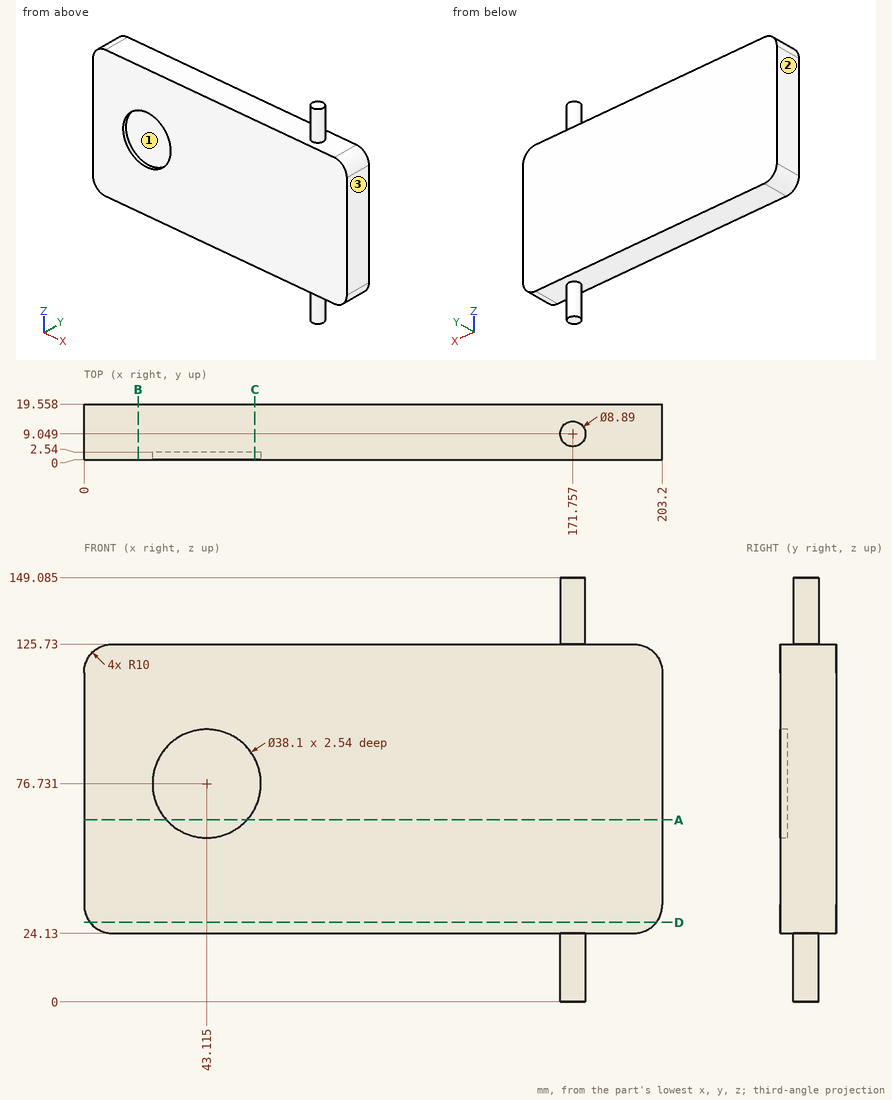
The drawing under review shows one solid part. Ordinate dimensions are in mm from its lowest x, y, z. Give positions to 0.01 mm unless a question says otherwise; leave off trailing zeros. Loops run counter-clockwise (first coordinate to the right, second up) from the corner with the lowest first, then second, coordinate; pieces in that order, holes last. Notation, with made-up numbers: M 21,-32 L 55,-32 A22 cw 55,-16 Z; hole C 88,-26 d5. An arc over 180 degrees is marked long. One line per question, with ' | ' between items. Start each with the question number.
1. To check wall thickness, follow L1, parallel to Z at x = 110, y = 8; L2, parallel to Z at x = 26, y = 2.25 (1 decimal); L3, parallel to X at y = 12.5, z = 140 (1 decimal). State the ranges of each line that lie inside material, in increasing order.
2. Add section A-A (z = 64). Write out the cut boundary in (x, y) (1 decimal).
3. Insertion check: P1, Ø6, axis at x = 109.5, y = 6.5, coming from the +Z side; P2, Ø10, axis at x = 112.5, y = 8.5, coming from the -Z side. Each pin has a flat end and moves straight along its axis. Give the tip position at first contact, or say it passes through.
4. Add section D-D (z = 28). Write out the cut boundary in (x, y), plus the area to 3 significant figures.
5. The part is to be moulded in two halves that separate along X. For the marked faces 1, 2 and 3, say which applies: released by +X, released by -X, zero draft, split by the parting line, or undercut.
6. Add section B-B (x = 19). Write out the cut boundary in (y, z).
7. Add section C-C (x = 60). Write out the cut boundary in (y, z), plus the area to 3 significant figures.
Worked out:
1) L1: z = 24.13 to 125.73 | L2: z = 24.1 to 68.4, 85.1 to 125.7 | L3: x = 169 to 174.6
2) outline: M 0,0 L 28.9,0 L 28.9,2.5 L 57.3,2.5 L 57.3,0 L 203.2,0 L 203.2,19.6 L 0,19.6 Z
3) P1: stops at z = 125.73 | P2: stops at z = 24.13
4) outline: M 2.1,0 L 201.1,0 L 201.1,19.56 L 2.1,19.56 Z | area: 3,890 mm²
5) face 1: undercut | face 2: released by -X | face 3: released by +X
6) outline: M 0,24.13 L 19.56,24.13 L 19.56,125.73 L 0,125.73 Z
7) outline: M 0,24.13 L 19.56,24.13 L 19.56,125.73 L 0,125.73 L 0,85.55 L 2.54,85.55 L 2.54,67.91 L 0,67.91 Z | area: 1,940 mm²
